Read the model definition and answer for the solid it produces. Units are mm, in the model's axes. Face numbers are marked on the shaded views. Round coordinates to 2 decimals unless told otherwise and drop trailing zeros. Write each loop counter-clockwise with the first axis right and the second up, starting at its lowest first coordinate (ties: lowest second). Pieces come first, ordered by that corner, then holes.
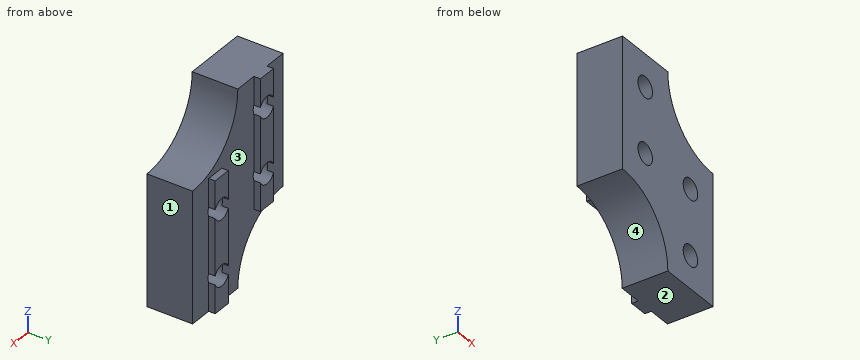
from build123d import *

# Parameters (mm, degrees)
MAIN_DEPTH                = 10
ESQUISSE2_R               = 1.6
TOPHOLE_DEPTH             = 14.747727085
LPATTERN1_COUNT           = 2
LPATTERN1_PITCH           = 10
LPATTERN2_COUNT           = 2
LPATTERN2_PITCH           = 10
LPATTERN2_2_COUNT         = 2
LPATTERN2_2_PITCH         = 10
LPATTERN3_COUNT           = 2
LPATTERN3_PITCH           = 10
LPATTERN3_COPY_1_DEPTH    = 10
LPATTERN3_COPY_2_SKETCH_R = 1.6
LPATTERN3_COPY_2_DEPTH    = 14.747727085
LPATTERN3_COPY_3_DEPTH    = 10
SKETCH1_W                 = 10
SKETCH1_H                 = 10
CUT_EXTRUDE1_DEPTH        = 27.248809497
FILLET1_R                 = 10
SKETCH2_W                 = 10
SKETCH2_H                 = 10
CUT_EXTRUDE2_DEPTH        = 1


with BuildPart() as part:
    # Esquisse1 → Main (new body)
    with BuildSketch(Plane.XY):
        Polygon((-5, 0), (-5, 7), (-1.45, 7), (-1.45, 8), (1.45, 8), (1.45, 7), (5, 7), (5, 0), align=None)
    main = extrude(amount=MAIN_DEPTH)

    # Esquisse2 → TopHole (cut, through all)
    with BuildSketch(Plane(origin=(0, 8, 0), x_dir=(1, 0, 0), z_dir=(0, 1, 0))):
        with Locations(Location((0, -5, 0), (0, 0, 270))):
            Circle(ESQUISSE2_R)
    tophole = extrude(amount=-TOPHOLE_DEPTH, mode=Mode.SUBTRACT)


with BuildPart() as lpattern1_1:
    # LPattern1: pattern copy
    add(part.part.moved(Location(Vector(0, 0, -1) * (1 * LPATTERN1_PITCH))))


with BuildPart() as part_1:
    add(part.part)

    add(lpattern1_1.part)  # LPattern2 merges LPattern1_1
    # LPattern2: Main ×2
    with Locations(*[(-i * LPATTERN2_PITCH, 0, 0) for i in range(1, LPATTERN2_COUNT)]):
        add(main)

    # LPattern2 2: TopHole ×2
    with Locations(*[(-i * LPATTERN2_2_PITCH, 0, 0) for i in range(1, LPATTERN2_2_COUNT)]):
        add(tophole, mode=Mode.SUBTRACT)

    # LPattern3: TopHole ×2
    with Locations(*[(0, 0, i * LPATTERN3_PITCH) for i in range(1, LPATTERN3_COUNT)]):
        add(tophole, mode=Mode.SUBTRACT)

    # LPattern3 copy 1 sketch → LPattern3 copy 1 (add)
    with BuildSketch(Plane(origin=(-10, 0, 10), x_dir=(1, 0, 0), z_dir=(0, 0, 1))):
        Polygon((-5, 0), (-5, 7), (-1.45, 7), (-1.45, 8), (1.45, 8), (1.45, 7), (5, 7), (5, 0), align=None)
    extrude(amount=LPATTERN3_COPY_1_DEPTH)

    # LPattern3 copy 2 sketch → LPattern3 copy 2 (cut, through all)
    with BuildSketch(Plane(origin=(-10, 8, 10), x_dir=(1, 0, 0), z_dir=(0, 1, 0))):
        with Locations(Location((0, -5, 0), (0, 0, 270))):
            Circle(LPATTERN3_COPY_2_SKETCH_R)
    extrude(amount=-LPATTERN3_COPY_2_DEPTH, mode=Mode.SUBTRACT)

    # LPattern3 copy 3 sketch → LPattern3 copy 3 (add)
    with BuildSketch(Plane.XY.offset(10)):
        Polygon((-5, 0), (-5, 7), (-1.45, 7), (-1.45, 8), (1.45, 8), (1.45, 7), (5, 7), (5, 0), align=None)
    extrude(amount=LPATTERN3_COPY_3_DEPTH)

    # Sketch1 → Cut-Extrude1 (cut, through all)
    with BuildSketch(Plane(origin=(0, 8, 0), x_dir=(1, 0, 0), z_dir=(0, 1, 0))):
        with Locations((0, -15)):
            Rectangle(SKETCH1_W, SKETCH1_H)
    extrude(amount=-CUT_EXTRUDE1_DEPTH, mode=Mode.SUBTRACT)

    # Fillet1
    fillet1_edges = [part_1.edges().sort_by_distance(p)[0] for p in [
        (-5, 3.5, 0),
        (-5, 3.5, 10),
    ]]
    fillet(fillet1_edges, radius=FILLET1_R - 0.0001)  # a hair under: the kernel refuses the full size

    # Sketch2 → Cut-Extrude2 (cut)
    with BuildSketch(Plane(origin=(0, 8, 0), x_dir=(1, 0, 0), z_dir=(0, 1, 0))):
        with Locations((-10, 5)):
            Rectangle(SKETCH2_W, SKETCH2_H)
        with Locations((0, -15)):
            Rectangle(SKETCH2_W, SKETCH2_H)
    extrude(amount=-CUT_EXTRUDE2_DEPTH, mode=Mode.SUBTRACT)


solid = part_1.part
Q1. Section B-B (y = 3) is taken. State how many separate pieces and enclosed holes the cut face has, then the cut area to 3 significant figures.
Verdict:
separate pieces: 1
enclosed holes: 4
area: 411 mm2
Q2. Section D-D (z = -4) is taken. Determine the outline of the cut face in (x, y).
Verdict:
outline: (-7, 0) - (-1.25, 0) - (-1.25, 8) - (-1.45, 8) - (-1.45, 7) - (-7, 7) - close; (1.25, 0) - (5, 0) - (5, 7) - (1.45, 7) - (1.45, 8) - (1.25, 8) - close
Q3. Determine the mould class of the marked faces 1, 2, 3 and 4 for opening direction X: pulls with the +X half, pulls with the -X half, needs draft (parallel to the pull), parting line crosses it, or undercut.
Verdict:
face 1: pulls with the +X half
face 2: needs draft
face 3: undercut
face 4: pulls with the -X half
Q4. Flat-ended cylindrical pins translate along their axes: pin 1 Ø0.5 at (y, z) = (7.5, 7) entering from -X; pin 2 Ø0.5 at (y, z) = (7.5, 3) entering from +X; pin 3 Ø0.5 at (x, y) = (-9.5, 7.5) entering from -Z. Find the tip coordinate at first contact, or state that the pin passes through.
Verdict:
pin 1: stops at x = -11.45
pin 2: stops at x = 1.45
pin 3: stops at z = 0
Q5. Section C-C (x = -10) is taken. Determine the outline of the cut face in (y, z).
Verdict:
outline: (0, -1.34) - (7, -1.34) - (7, 0) - (8, 0) - (8, 3.4) - (0, 3.4) - close; (0, 6.6) - (8, 6.6) - (8, 13.4) - (0, 13.4) - close; (0, 16.6) - (8, 16.6) - (8, 20) - (0, 20) - close
Q6. Straight lines are drawn through the part: probe 1 along X at (y, z) = (2.75, 5); probe 2 along Z at (x, y) = (-0.5, 4); probe 3 along Z at (x, y) = (0, 4). For each, find the intervals that lie inside material, in ascending order.
Verdict:
probe 1: x = -15 to -11.6, -8.4 to -1.6, 1.6 to 5
probe 2: z = -10 to -6.52, -3.48 to 3.48, 6.52 to 11.65
probe 3: z = -10 to -6.6, -3.4 to 3.4, 6.6 to 11.34
Q7. Section A-A (z = 5) is taken. Determine the outline of the cut face in (x, y), then the cut area to 3 significant figures.
Verdict:
outline: (-15, 0) - (-11.6, 0) - (-11.6, 7) - (-15, 7) - close; (-8.4, 0) - (-1.6, 0) - (-1.6, 7) - (-8.4, 7) - close; (1.6, 0) - (5, 0) - (5, 7) - (1.6, 7) - close
area: 95.2 mm2
